The listing builds one solid part. Answer for the finished solid, in the listing's coordinates (mm). Face numbers are marked on the shaded views. A direction names the side the tool comes from. Coordinates: 2 decimals unless noted, no trailing zeros. Order: outer loops, then holes, each group sorted by start corner. A loop starts at its lowest first (then second) coordinate and runs counter-clockwise, first axis right, second up.
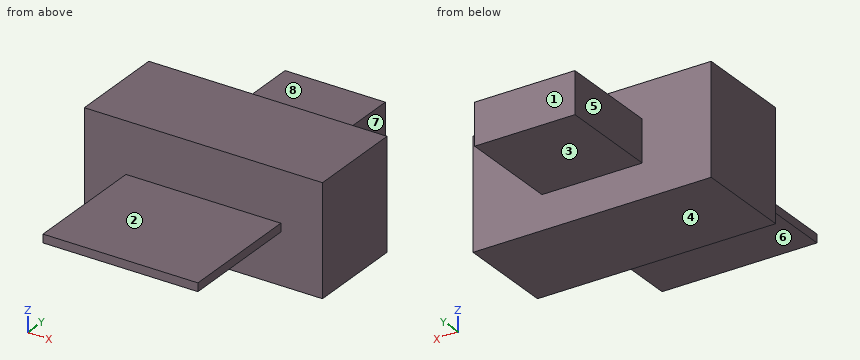
from build123d import *

# Parameters (mm, degrees)
SKETCH_1_W      = 8.55
SKETCH_1_H      = 3.5
EXTRUDE_1_DEPTH = 3.95
SKETCH_2_W      = 3.6
SKETCH_2_H      = 1.5
EXTRUDE_2_DEPTH = 3.65
SKETCH_3_W      = 5.56
SKETCH_3_H      = 0.3
EXTRUDE_3_DEPTH = 4.5


with BuildPart() as part:
    # 草图1 → 凸台-拉伸1 (new body)
    with BuildSketch(Plane.XY):
        with Locations((4.275, 1.75)):
            Rectangle(SKETCH_1_W, SKETCH_1_H)
    extrude(amount=EXTRUDE_1_DEPTH)

    # 草图2 → 凸台-拉伸2 (add)
    with BuildSketch(Plane(origin=(0, 3.5, 0), x_dir=(1, 0, 0), z_dir=(0, 1, 0))):
        with Locations((4.275, -1.975)):
            Rectangle(SKETCH_2_W, SKETCH_2_H)
    extrude(amount=EXTRUDE_2_DEPTH)

    # 草图3 → 凸台-拉伸3 (add)
    with BuildSketch(Plane.XZ):
        with Locations((4.275, 1.975)):
            Rectangle(SKETCH_3_W, SKETCH_3_H)
    extrude(amount=EXTRUDE_3_DEPTH)


solid = part.part
1) Consider L1, parallel to X at y = 5, z = 1.4 (3 decimals); L2, parallel to Y at x = 1, z = 1.95; L3, parallel to Y at x = 4.25, z = 1.35. Determine where each line is inside the solid, lowest interval first.
2) Section D-D (x = 2.25) is taken. Give the vertices of the cut face in (y, z) (3 decimals).
3) A tool of negligible diameter and unlimited length cuts with its end or side. For the marked faces 4, 5, 6, 7 and 8, from which of +Z, -Z, +X, -X, +Y, -Y can it reach the whole face along a straight path? Write none if from no direction.
4) Section C-C (y = -2.25) is taken. Give the vertices of the cut face in (x, z) (3 decimals), then the cut area to 3 significant figures.
5) Each of these flat-tipped pins is pushed along its axis until it touches: P1, Ø3.5, axis at x = 5, y = -2.5, coming from the -Z side (3 decimals); P2, Ø4, axis at x = 5, y = 6, coming from the -Z side (3 decimals); P3, Ø0.8, axis at y = 5, z = 2, coming from the -X side (3 decimals). Where does it stop, or does it pass through?
6) Section A-A (z = 2) is taken. Give the vertices of the cut face in (x, y) (3 decimals), then the cut area to 3 significant figures.
7) Section B-B (x = 5.5) is taken. Give the vertices of the cut face in (y, z) (3 decimals), then the cut area to 4 significant figures.
8) Determine the mould class of the marked faces 1, 2 and 3 for opening direction Z: released by +Z, released by -Z, zero draft, split by the parting line, or undercut.
Filled sheet:
1. L1: x = 2.475 to 6.075
1. L2: y = 0 to 3.5
1. L3: y = 0 to 7.15
2. outline: (-4.5, 1.825) - (0, 1.825) - (0, 0) - (3.5, 0) - (3.5, 3.95) - (0, 3.95) - (0, 2.125) - (-4.5, 2.125) - close
3. face 4: -Z, +X, -X, +Y, -Y
3. face 5: +Z, -Z, -X, +Y
3. face 6: -Z, +X, -X, -Y
3. face 7: +Z, -Z, +X, +Y
3. face 8: +Z, +X, -X, +Y
4. outline: (1.495, 1.825) - (7.055, 1.825) - (7.055, 2.125) - (1.495, 2.125) - close
4. area: 1.67 mm2
5. P1: stops at z = 1.825
5. P2: stops at z = 1.225
5. P3: stops at x = 2.475
6. outline: (0, 0) - (1.495, 0) - (1.495, -4.5) - (7.055, -4.5) - (7.055, 0) - (8.55, 0) - (8.55, 3.5) - (6.075, 3.5) - (6.075, 7.15) - (2.475, 7.15) - (2.475, 3.5) - (0, 3.5) - close
6. area: 68.1 mm2
7. outline: (-4.5, 1.825) - (0, 1.825) - (0, 0) - (3.5, 0) - (3.5, 1.225) - (7.15, 1.225) - (7.15, 2.725) - (3.5, 2.725) - (3.5, 3.95) - (0, 3.95) - (0, 2.125) - (-4.5, 2.125) - close
7. area: 20.65 mm2
8. face 1: zero draft
8. face 2: released by +Z
8. face 3: released by -Z
